Here's the drawing with two shaded views (mm, measured from the low corner). I have some questions. Coordinates: 2 decimals unless noted, no trailing zeros. Write each loop counter-clockwise with the first axis right and the second up, starting at its lowest first coordinate (ties: lowest second). Pieces come first, ordered by that corner, then holes.
Item 1: For P1, Ø12, axis at y = 6, z = 24.5, coming from the -X side; P2, Ø2, axis at x = 8.5, z = 64.5, coming from the -Y side, each with a flat end and sliding along its axis, tell me the tip position at first contact or that it passes through.
Item 2: If I drill on probe 1 along Z at (x, y) = (44.5, 11); probe 2 along Z at (x, y) = (40.5, 49.1); probe 3 along Z at (x, y) = (49, 25), over which ranges is the centre line in solid material (lowest first)?
Item 3: I want a section at B-B on x = 9.5. Please give me the cut outline in (y, z), then the cut area to 3 significant figures.
Item 4: I want a section at C-C on y = 42. Please give me the cut outline in (x, z).
Item 5: I want a section at D-D on x = 25. Please give me the cut outline in (y, z).
Item 6: Thinking about a two-plate mould opening in Z: for the marked faces 1, 2, 3 and 4, which applies, +Z half, -Z half, draft (parallel to the pull), parting line (faces both ways), or undercut?
Item 7: I want a section at A-A on z = 60. Please give me the cut outline in (x, y), then the cut area to 4 significant figures.
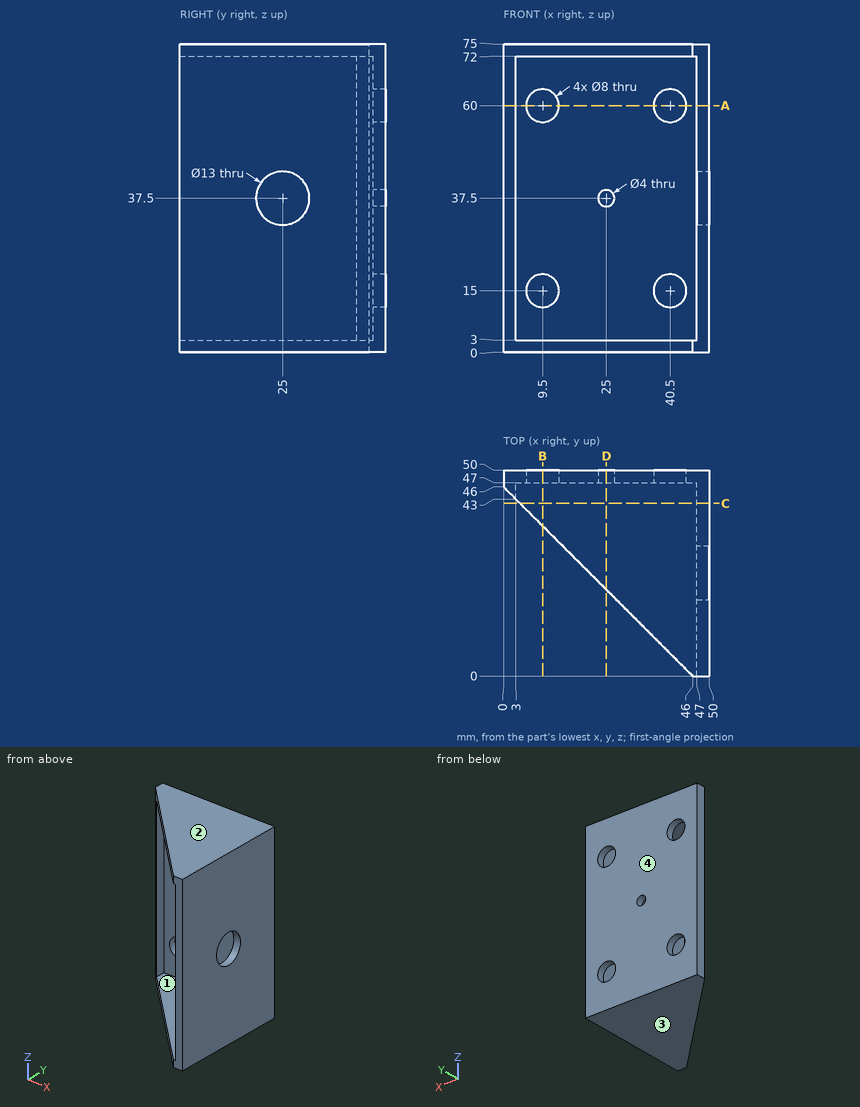
Response values:
1. P1: stops at x = 47
1. P2: stops at y = 47
2. probe 1: z = 0 to 3, 72 to 75
2. probe 2: z = 0 to 11, 19 to 56, 64 to 75
2. probe 3: z = 0 to 31, 44 to 75
3. outline: (36.5, 0) - (50, 0) - (50, 11) - (47, 11) - (47, 3) - (36.5, 3) - close; (36.5, 72) - (47, 72) - (47, 64) - (50, 64) - (50, 75) - (36.5, 75) - close; (47, 19) - (50, 19) - (50, 56) - (47, 56) - close
3. area: 240 mm2
4. outline: (4, 0) - (50, 0) - (50, 75) - (4, 75) - (4, 72) - (47, 72) - (47, 3) - (4, 3) - close
5. outline: (21, 0) - (50, 0) - (50, 35.5) - (47, 35.5) - (47, 3) - (21, 3) - close; (21, 72) - (47, 72) - (47, 39.5) - (50, 39.5) - (50, 75) - (21, 75) - close
6. face 1: undercut
6. face 2: +Z half
6. face 3: -Z half
6. face 4: draft
7. outline: (0, 46) - (3, 43) - (3, 47) - (5.5, 47) - (5.5, 50) - (0, 50) - close; (13.5, 47) - (36.5, 47) - (36.5, 50) - (13.5, 50) - close; (44.5, 47) - (47, 47) - (47, 0) - (50, 0) - (50, 50) - (44.5, 50) - close
7. area: 250.5 mm2
